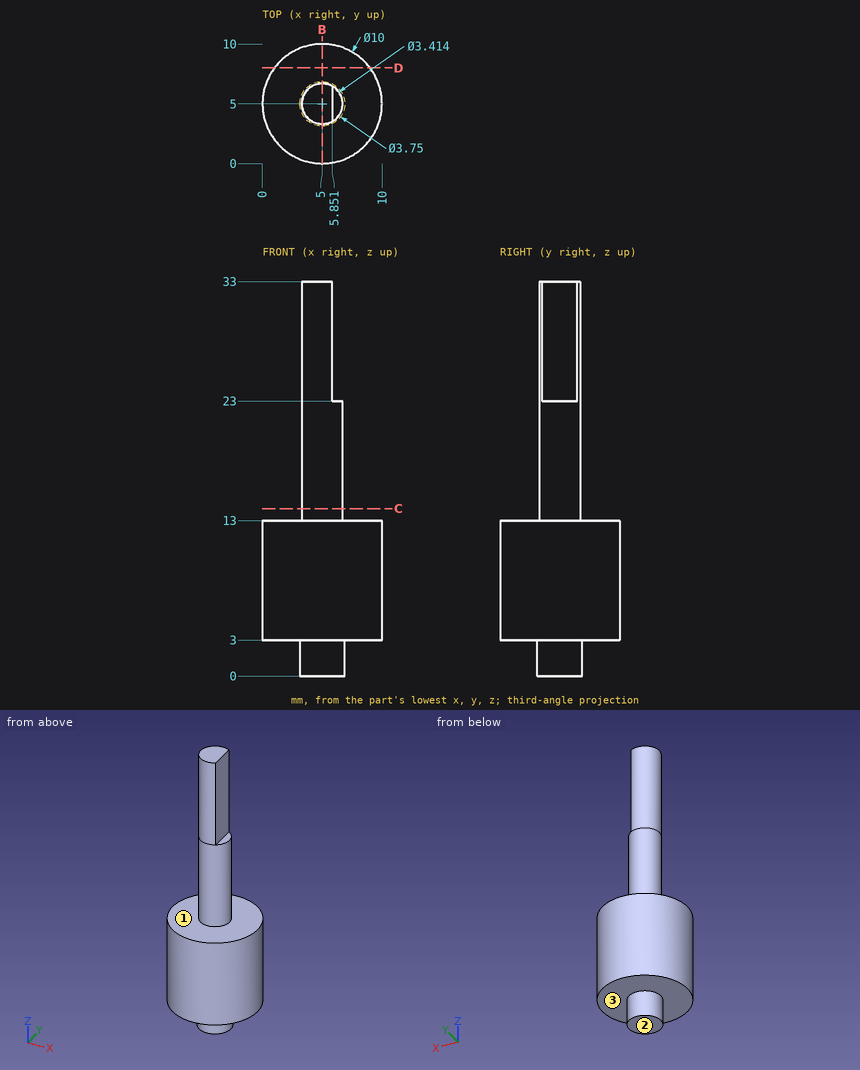
Source: three-view drawing plus pictorial views. Frame: mm from the lowest corner of the part. A direction names the side the tool comes from. Round coordinates to 2 decimals unless told otherwise and drop trailing zeros. Loops run counter-clockwise (first coordinate to the right, second up) from the corner with the lowest first, then second, coordinate; pieces in that order, holes last. Notation, with made-up numbers: M 76.5,62.25 L 133.5,62.25 A24 ccw 133.5,93.25 Z; hole C -22.5,47.25 d5. An arc over 180 degrees is marked long. Answer as CSV lines item,"result". Start each with the question number.
(1) Section C-C, the plane z = 14. Output: boundary loops of the cut face in (x, y).
(2) Reachability of the marked faces 1, 2 and 3 from +Z, -Z, +X, -X, +Y, -Y: full face, straight path, thin tool, end or side. Return the list, or none.
(3) Section B-B, the plane x = 5. Output: boundary loops of the cut face in (y, z) (1 decimal).
(4) First-contact query: pin 1 (1 mm diameter, centred on x = 4, z = 29.5, fed in from -Y); pin 2 (1.5 mm diameter, centred on y = 7.5, z = 26.5, fed in from -X); pin 3 (1 mm diameter, centred on y = 1, z = 8, fed in from +X); pin 4 (0.9 mm diameter, centred on y = 4.5, z = 26, fed in from +X). Flat tips, straight axial feed; report the tip coordinate or a pass-through.
(5) Line query: line 1 (Z direction, x = 2.75, y = 6.5); line 2 (X direction, y = 4.75, z = 8.5); line 3 (Y direction, x = 4, z = 21.5) (1 decimal). Output: solid intervals per line, ascending. Write a range as [from, to].
(6) Section D-D, the plane y = 8. Output: boundary loops of the cut face in (x, z).
Values found:
1,outline,"C 5,5 d3.41"
2,face 1,"+Z"
2,face 2,"-Z, +X, -X, +Y, -Y"
2,face 3,"-Z"
3,outline,"M 0,3 L 3.1,3 L 3.1,0 L 6.9,0 L 6.9,3 L 10,3 L 10,13 L 6.7,13 L 6.7,33 L 3.3,33 L 3.3,13 L 0,13 Z"
4,pin 1,"stops at y = 3.37"
4,pin 2,"passes through"
4,pin 3,"stops at x = 8.57"
4,pin 4,"stops at x = 5.85"
5,line 1,"z = [3, 13]"
5,line 2,"x = [0.01, 9.99]"
5,line 3,"y = [3.6, 6.4]"
6,outline,"M 1,3 L 9,3 L 9,13 L 1,13 Z"
